from build123d import *

# Parameters (mm, degrees)
SKETCH3_R               = 19.05
CUT_EXTRUDE1_DEPTH      = 26.4
CUT_EXTRUDE1_DEPTH_BACK = 26.4
SKETCH4_W               = 14.478
SKETCH4_H               = 4.572
CUT_EXTRUDE3_DEPTH      = 30.988
CIRPATTERN2_COUNT       = 4


with BuildPart() as part:
    # Sketch2 → Revolve1 (revolve)
    with BuildSketch(Plane.XY):
        with BuildLine():
            Line((0, 0), (0, 137.668))
            Line((0, 137.668), (-12.7, 137.668))
            Line((-12.7, 137.668), (-12.7, 47.397045256))
            ThreePointArc((-12.7, 47.397045256), (-24.534515988, 18.825996254), (0, 0))
        make_face()
    revolve(axis=Axis((0, 0, 0), (0, 1, 0)))

    # Sketch3 → Cut-Extrude1 (cut, two sides)
    with BuildSketch(Plane.XY) as cut_extrude1_sk:
        with Locations((0, 25.4)):
            Circle(SKETCH3_R)
    extrude(amount=CUT_EXTRUDE1_DEPTH, mode=Mode.SUBTRACT)
    extrude(cut_extrude1_sk.sketch, amount=-CUT_EXTRUDE1_DEPTH_BACK, mode=Mode.SUBTRACT)

    # Sketch4 → Cut-Extrude3 (cut)
    with BuildSketch(Plane(origin=(0, 137.668, 0), x_dir=(1, 0, 0), z_dir=(0, 1, 0))):
        with Locations((0, 12.720887589)):
            Rectangle(SKETCH4_W, SKETCH4_H)
    cut_extrude3 = extrude(amount=-CUT_EXTRUDE3_DEPTH, mode=Mode.SUBTRACT)

    # CirPattern2: Cut-Extrude3 ×4 about axis
    cirpattern2_axis = Axis((0, 0, 0), (0, 1, 0))
    for i in range(1, CIRPATTERN2_COUNT):
        add(cut_extrude3.rotate(cirpattern2_axis, i * 360 / CIRPATTERN2_COUNT), mode=Mode.SUBTRACT)


solid = part.part
Here's how the part is built. I have some questions about the finished solid (model axes, mm). A direction names the side the tool comes from. Round coordinates to 2 decimals unless told otherwise and drop trailing zeros. Write each loop counter-clockwise with the first axis right and the second up, starting at its lowest first coordinate (ties: lowest second). Pieces come first, ordered by that corner, then holes. Notation, with made-up numbers: (44, 83) -> (92, 83) arc R11 ccw to (92, 89) -> close; hole circle Ø5 at (2, 89.5). An arc over 180 degrees is marked (long way). One line per item, written item: value.
1) Suppose I cut it at C-C on y = 81. List the corners of the cut face in (x, z) for me.
Filled sheet:
outline: circle Ø25.4 at (0, 0)
2) I'm going to push flat-ended pins straight in: pin 1 Ø1.1 at (x, z) = (12, 3.5) entering from +Y; pin 2 Ø7 at (y, z) = (125.5, 2.5) entering from -X; pin 3 Ø1 at (x, z) = (-20, -10) entering from +Y. Where does each tip first touch, or does it pass through?
Filled sheet:
pin 1: stops at y = 106.68
pin 2: stops at x = -10.43
pin 3: stops at y = 38.33
3) If I drill on line 1 (X direction, y = 123, z = -5); line 2 (X direction, y = 25, z = 8); line 3 (X direction, y = 14, z = 10.5), over which ranges is the centre line in solid material (lowest first)? Write a range as [from, to].
Filled sheet:
line 1: x = [-10.43, 10.43]
line 2: x = [-24.1, -19.05], [19.05, 24.1]
line 3: x = [-20.12, -15.26], [15.26, 20.12]
4) Suppose I cut it at D-D on z = -9. List the corners of the cut face in (x, y) for me.
Filled sheet:
outline: (-8.96, 47.4) arc R23.75 ccw (long way) to (8.96, 47.4) -> (8.96, 137.67) -> (-8.96, 137.67) -> close; hole circle Ø38.1 at (0, 25.4)
5) For faces 1 (the face through (0, 122, -10.435)), 2 (the face through (0, 106.68, 11)), 3 (the face through (10.435, 122, 0)), 4 (the face through (12.688, 81.871, 0.558)), 5 (the face through (-11, 106.68, 0)), which set-ups out of +Z, -Z, +X, -X, +Y, -Y let a thin tool reach every point of the face, with its end or its side?
Filled sheet:
face 1: -Z, +X, -X, +Y
face 2: +Z, +X, -X, +Y
face 3: +Z, -Z, +X, +Y
face 4: +Y
face 5: +Z, -Z, -X, +Y
6) Suppose I cut it at B-B on y = 25.4. List the corners of the cut face in (x, z) for me, plus the area to 3 significant figures.
Filled sheet:
outline: (-19.05, -16.8) -> (-19.05, 16.8) arc R25.4 ccw to start; (19.05, -16.8) arc R25.4 ccw to (19.05, 16.8) -> close
area: 292 mm2
7) Suppose I cut it at A-A on x = 0. List the corners of the cut face in (y, z) for me.
Filled sheet:
outline: (6.35, -16.8) -> (6.35, 16.8) arc R25.4 ccw to start; (44.45, -16.8) arc R25.4 ccw to (47.4, -12.7) -> (106.68, -12.7) -> (106.68, -10.43) -> (137.67, -10.43) -> (137.67, 10.43) -> (106.68, 10.43) -> (106.68, 12.7) -> (47.4, 12.7) arc R25.4 ccw to (44.45, 16.8) -> close
